CAD build for the part. Positions are in the model's coordinates, mm. A direction names the side the tool comes from. Coordinates: 2 decimals unless noted, no trailing zeros. Loops run counter-clockwise (first coordinate to the right, second up) from the corner with the lowest first, then second, coordinate; pieces in that order, holes last. Notation, with made-up numbers: (-15.75, 26) -> (28.25, 26) arc R25 cw to (28.25, 44) -> close; hole circle Ø2 at (28.5, 67). An arc over 180 degrees is marked (long way). Write each question's results on one line, items separated by ' | '.
```python
from build123d import *

# Parameters (mm, degrees)
SKETCH1_R           = 65
SKETCH1_R_2         = 1.5
BOSS_EXTRUDE1_DEPTH = 4.75
SKETCH3_W           = 10
SKETCH3_H           = 5
CUT_EXTRUDE1_DEPTH  = 5
SKETCH4_R           = 1.5
CUT_EXTRUDE2_DEPTH  = 93.012567223
CUT_EXTRUDE3_DEPTH  = 93.012567223


with BuildPart() as part:
    # Sketch1 → Boss-Extrude1 (new body)
    with BuildSketch(Plane(origin=(0, 0, 0), x_dir=(1, 0, 0), z_dir=(0, 1, 0))):
        with Locations(Location((0, 0, 0), (0, 0, 270))):
            Circle(SKETCH1_R)
        with Locations(Location((0, -57.5, 0), (0, 0, 270))):
            Circle(SKETCH1_R_2, mode=Mode.SUBTRACT)
        with Locations(Location((40.658639918, -40.658639918, 0), (0, 0, 270))):
            Circle(SKETCH1_R_2, mode=Mode.SUBTRACT)
        with Locations(Location((40.658639918, 40.658639918, 0), (0, 0, 270))):
            Circle(SKETCH1_R_2, mode=Mode.SUBTRACT)
        with Locations(Location((0, 57.5, 0), (0, 0, 90))):
            Circle(SKETCH1_R_2, mode=Mode.SUBTRACT)
        with Locations(Location((-40.658639918, 40.658639918, 0), (0, 0, 90))):
            Circle(SKETCH1_R_2, mode=Mode.SUBTRACT)
        with Locations(Location((-40.658639918, -40.658639918, 0), (0, 0, 90))):
            Circle(SKETCH1_R_2, mode=Mode.SUBTRACT)
        with BuildLine():
            ThreePointArc((44.349781873, 7.622128822), (-45, 0), (44.349781873, -7.622128822))
            add(Edge.make_bspline(
                [(44.349781873, -7.622128822), (45, -0.795007083), (39.088787829, 0)],
                knots=[0, 0, 0, 1, 1, 1], degree=2))
            add(Edge.make_bspline(
                [(44.349781873, 7.622128822), (45, 0.795007083), (39.088787829, 0)],
                knots=[0, 0, 0, 1, 1, 1], degree=2))
        make_face(mode=Mode.SUBTRACT)
    extrude(amount=BOSS_EXTRUDE1_DEPTH)

    # Sketch3 → Cut-Extrude1 (cut)
    with BuildSketch(Plane(origin=(0, 4.75, 0), x_dir=(1, 0, 0), z_dir=(0, 1, 0))):
        with Locations((61.25, 0)):
            Rectangle(SKETCH3_W, SKETCH3_H)
        with Locations((-61.25, 0)):
            Rectangle(SKETCH3_W, SKETCH3_H)
    extrude(amount=-CUT_EXTRUDE1_DEPTH, mode=Mode.SUBTRACT)

    # Sketch4 → Cut-Extrude2 (cut, through all)
    with BuildSketch(Plane(origin=(0, 4.75, 0), x_dir=(1, 0, 0), z_dir=(0, 1, 0))):
        with Locations(Location((54.951905284, -9.5, 0), (0, 0, 270))):
            Circle(SKETCH4_R)
        with Locations(Location((-54.951905284, -9.5, 0), (0, 0, 90))):
            Circle(SKETCH4_R)
    extrude(amount=-CUT_EXTRUDE2_DEPTH, mode=Mode.SUBTRACT)

    # Sketch5 → Cut-Extrude3 (cut, through all)
    with BuildSketch(Plane(origin=(0, 4.75, 0), x_dir=(1, 0, 0), z_dir=(0, 1, 0))):
        with BuildLine():
            Line((-64.951905284, 2.5), (-56.25, 2.5))
            Line((-56.25, 2.5), (-56.25, 32.572035552))
            ThreePointArc((-56.25, 32.572035552), (-62.438428004, 18.067725599), (-64.951905284, 2.5))
        make_face()
        with BuildLine():
            ThreePointArc((64.951905284, 2.5), (62.438428004, 18.067725599), (56.25, 32.572035552))
            Line((56.25, 32.572035552), (56.25, 2.5))
            Line((56.25, 2.5), (64.951905284, 2.5))
        make_face()
    extrude(amount=-CUT_EXTRUDE3_DEPTH, mode=Mode.SUBTRACT)


solid = part.part
```
Q1. Cut at D-D on y = 1.45. Give the number of separate pieces and of enclosed holes in the cut face, and give its area (3 significant figures).
Results are:
separate pieces: 1 | enclosed holes: 9 | area: 6,450 mm^2
Q2. Cut at C-C on z = 9.5. Write the cut outline in (x, y).
Results are:
outline: (-64.3, 0) -> (-56.45, 0) -> (-56.45, 4.75) -> (-64.3, 4.75) -> close; (-53.45, 0) -> (-43.99, 0) -> (-43.99, 4.75) -> (-53.45, 4.75) -> close; (43.99, 0) -> (53.45, 0) -> (53.45, 4.75) -> (43.99, 4.75) -> close; (56.45, 0) -> (64.3, 0) -> (64.3, 4.75) -> (56.45, 4.75) -> close
Q3. Drop flat-ended pins along their axis: pin 1 (1.4 mm diameter, centred on y = 3.5, z = -8.5, fed in from -X); pin 2 (1.4 mm diameter, centred on y = 3, z = -7, fed in from +X). Give the stop position or say it passes through.
Results are:
pin 1: x = -56.25 | pin 2: x = 56.25
Q4. Which spindle directions (+Z, -Z, +X, -X, +Y, -Y) get a long thin tool onto all of the face, cutting with end or side? Do faces 5 (the flat face through (-61, 2, 2.5)), 6 (the cylindrical face through (-39.75, 2.34, 41.85)), 7 (the flat face through (61, 2, 2.5)). Say none if no direction does.
Results are:
face 5: -Z, -X, +Y, -Y | face 6: +Y, -Y | face 7: -Z, +X, +Y, -Y
Q5. Pull direction X, two halves, no side cores. Call faces 1 (the cylindrical face through (56.44, 2.41, 9.3)), 2 (the flat face through (56.25, 2, -15)), 3 (the cylindrical face through (-39.746, 2.342, -39.468)), 4 (the flat face through (39, 0, 24)): +X half, -X half, draft (parallel to the pull), parting line (faces both ways), or undercut.
Results are:
face 1: undercut | face 2: +X half | face 3: undercut | face 4: draft
Q6. Cut at A-A on x = 0. Write the cut outline in (y, z), and give its area (4 significant figures).
Results are:
outline: (0, -65) -> (4.75, -65) -> (4.75, -59) -> (0, -59) -> close; (0, -56) -> (4.75, -56) -> (4.75, -45) -> (0, -45) -> close; (0, 45) -> (4.75, 45) -> (4.75, 56) -> (0, 56) -> close; (0, 59) -> (4.75, 59) -> (4.75, 65) -> (0, 65) -> close | area: 161.5 mm^2
Q7. Cut at B-B on z = -37. Write the cut outline in (x, y), and give its area (3 significant figures).
Results are:
outline: (-53.44, 0) -> (-25.61, 0) -> (-25.61, 4.75) -> (-53.44, 4.75) -> close; (25.61, 0) -> (53.44, 0) -> (53.44, 4.75) -> (25.61, 4.75) -> close | area: 264 mm^2
Q8. Wall check: L1, parallel to X at y = 4, z = 39.5; L2, parallel to X at y = 3.55, z = 27.5; L3, parallel to X at y = 4.5, z = -6. Give the ranges that are in metal, low to high. Write a range as from..to.
Results are:
L1: -51.62..-41.61, -39.71..-21.56, 21.56..39.71, 41.61..51.62 | L2: -58.9..-35.62, 35.62..58.9 | L3: -56.25..-44.6, 44.41..56.25
